```python
from build123d import *

# Parameters (mm, degrees)
SKETCH_1_R            = 13.25
SKETCH_1_R_2          = 4
EXTRUDE_288_DEPTH     = 8
SKETCH_2_R            = 2.65
EXTRUDE_567_DEPTH     = 4
SKETCH_3_R            = 5.95
SKETCH_3_R_2          = 4
EXTRUDE_693_DEPTH     = 4
SKETCH_4_R            = 1.5
CUT_EXTRUDE_831_DEPTH = 14.25
SKETCH_5_R            = 1.5
CUT_EXTRUDE_2_DEPTH   = 24.9


with BuildPart() as part:
    # 草图1 → Extrude 288 (new body)
    with BuildSketch(Plane(origin=(0, 0, 0), x_dir=(1, 0, 0), z_dir=(0, 1, 0))):
        Circle(SKETCH_1_R)
        Circle(SKETCH_1_R_2, mode=Mode.SUBTRACT)
    extrude(amount=EXTRUDE_288_DEPTH)

    # 草图2 → Extrude 567 (add)
    with BuildSketch(Plane(origin=(0, 0, 0), x_dir=(1, 0, 0), z_dir=(0, 1, 0))):
        with BuildLine():
            Line((-20.602876712, -5.136776341), (-5.517808219, -12.046422392))
            Line((-5.517808219, -12.046422392), (-5.517808219, 12.046422392))
            Line((-5.517808219, 12.046422392), (-20.602876712, 5.136776341))
            ThreePointArc((-20.602876712, 5.136776341), (-23.9, 0), (-20.602876712, -5.136776341))
        make_face()
        with Locations((-18.25, 0)):
            Circle(SKETCH_2_R, mode=Mode.SUBTRACT)
        with BuildLine():
            Line((20.602876712, 5.136776341), (5.517808219, 12.046422392))
            Line((5.517808219, 12.046422392), (5.517808219, -12.046422392))
            Line((5.517808219, -12.046422392), (20.602876712, -5.136776341))
            ThreePointArc((20.602876712, -5.136776341), (23.9, 0), (20.602876712, 5.136776341))
        make_face()
        with Locations((18.25, 0)):
            Circle(SKETCH_2_R, mode=Mode.SUBTRACT)
    extrude(amount=EXTRUDE_567_DEPTH)

    # 草图3 → Extrude 693 (add)
    with BuildSketch(Plane(origin=(0, 8, 0), x_dir=(1, 0, 0), z_dir=(0, 1, 0))):
        Circle(SKETCH_3_R)
        Circle(SKETCH_3_R_2, mode=Mode.SUBTRACT)
    extrude(amount=EXTRUDE_693_DEPTH)

    # 草图4 → Cut-Extrude 831 (cut, through all)
    with BuildSketch(Plane.XY):
        with Locations((0, 10)):
            Circle(SKETCH_4_R)
    extrude(amount=-CUT_EXTRUDE_831_DEPTH, mode=Mode.SUBTRACT)

    # 草图5 → 紧定2 (cut, through all)
    with BuildSketch(Plane(origin=(0, 0, 0), x_dir=(0, 0, -1), z_dir=(1, 0, 0))):
        with Locations((0, 10)):
            Circle(SKETCH_5_R)
    extrude(amount=-CUT_EXTRUDE_2_DEPTH, mode=Mode.SUBTRACT)


solid = part.part
```
Geometry check sheet. Reference: the model listing, model coordinates, mm. A direction names the side the tool comes from. Coordinates: 2 decimals unless noted, no trailing zeros. Write each loop counter-clockwise with the first axis right and the second up, starting at its lowest first coordinate (ties: lowest second). Pieces come first, ordered by that corner, then holes. Notation, with made-up numbers: M 26.25,-14 L 69.25,-14 A32 ccw 69.25,21 Z; hole C 18.5,18.5 d9. An arc over 180 degrees is marked long. One line per item, written item: value. Start each with the question number.
(1) Sectioned sample at B-B, the plane y = 11. Enter the section's corners in (x, z), and give its area (3 significant figures).
(2) Sectioned sample at D-D, the plane z = -8.5. Enter the section's corners in (x, y), and give its area (3 significant figures).
(3) Sectioned sample at C-C, the plane x = -19. Enter the section's corners in (y, z).
(4) Sectioned sample at A-A, the plane x = 0. Enter the section's corners in (y, z), and give its area (3 significant figures).
(5) Release check for a two-part mould opening along Y. For faces 1 (the face through (5, 0, 0)), 2 (the face through (-15.722, 1.972, -0.796)), 3 (the face through (6, 8, 3)), 4 (the face through (-4.813, 8.536, 0.325)) record: released by +Y, released by -Y, zero draft, split by the parting line, or undercut.
(6) Depth check by flat-ended pin: pin 1 (7 mm diameter, centred on x = -18.25, z = 0, fed in from +Y); pin 2 (3 mm diameter, centred on x = -15, y = 3, fed in from -Z); pin 3 (5.5 mm diameter, centred on x = -15.5, z = 0, fed in from +Y). Enter the tip coordinate at first touch or a pass-through.
(7) Scan lines: line 1 along X through (y, z) = (0.9, 0); line 2 along X through (y, z) = (7.5, 0). Record each from-to range of solid material in increasing order. Write a range as [from, to].
(8) Tool access check on faces 5 (the face through (5.496, 9.972, 2.279)), 6 (the face through (-0.325, 8.536, -4.816)), 7 (the face through (23.9, 2, 0.1)). Record the directions out of +Z, -Z, +X, -X, +Y, -Y that give a thin tool (end or side, any length) a straight path to the whole face; none if there is none.
Filled sheet:
1. outline: M -5.84,-1.12 A5.95 ccw -1.12,-5.84 L -1.12,-3.84 A4 cw -3.84,-1.12 Z; M -5.84,1.12 L -3.84,1.12 A4 cw long 1.12,-3.84 L 1.12,-5.84 A5.95 ccw long Z
1. area: 52.2 mm²
2. outline: M -13.26,0 L 13.26,0 L 13.26,4 L 10.16,4 L 10.16,8 L -10.16,8 L -10.16,4 L -13.26,4 Z
2. area: 187 mm²
3. outline: M 0,-5.87 L 4,-5.87 L 4,-2.54 L 0,-2.54 Z; M 0,2.54 L 4,2.54 L 4,5.87 L 0,5.87 Z
4. outline: M 0,-13.25 L 8,-13.25 L 8,-5.95 L 8.5,-5.95 L 8.5,-4 L 0,-4 Z; M 0,4 L 12,4 L 12,5.95 L 8,5.95 L 8,13.25 L 0,13.25 Z; M 11.5,-5.95 L 12,-5.95 L 12,-4 L 11.5,-4 Z
4. area: 158 mm²
5. face 1: released by -Y
5. face 2: zero draft
5. face 3: released by +Y
5. face 4: undercut
6. pin 1: y = 4
6. pin 2: z = -8.39
6. pin 3: y = 8
7. line 1: [-23.9, -20.9], [-15.6, -4], [4, 15.6], [20.9, 23.9]
7. line 2: [-13.25, -4], [4, 13.25]
8. face 5: +Y
8. face 6: -Z
8. face 7: +X, +Y, -Y
